```python
from build123d import *

# Parameters (mm, degrees)
F1_DEPTH = 1524
F3_DEPTH = 25.4
F5_DEPTH = 25.4


with BuildPart() as f1:
    # F0 (on Front) → F1 (new body)
    with BuildSketch(Plane.XZ):
        Polygon((-50.705169, 29.967905), (-53.880169, 29.967905), (-53.880169, -14.482095), (-9.430169, -14.482095), (-9.430169, -11.307095), (-50.705169, -11.307095), align=None)
    extrude(amount=F1_DEPTH)

    # F2 (on face) → F3 (cut)
    with BuildSketch(Plane.XY.offset(-11.307095)):
        Polygon((-50.705169, 0), (-9.430169, -41.340452), (-9.430169, 0), align=None)
    extrude(amount=-F3_DEPTH, mode=Mode.SUBTRACT)

    # F4 (on face) → F5 (cut)
    with BuildSketch(Plane.XY.offset(-11.307095)):
        Polygon((-9.430169, -1524), (-9.430169, -1482.725), (-50.705169, -1524), align=None)
    extrude(amount=-F5_DEPTH, mode=Mode.SUBTRACT)


solid = f1.part
```
Here's how the part is built. I have some questions about the finished solid (model axes, mm). A direction names the side the tool comes from. Round coordinates to 2 decimals unless told otherwise and drop trailing zeros. Loops run counter-clockwise (first coordinate to the right, second up) from the corner with the lowest first, then second, coordinate; pieces in that order, holes last.
1. Suppose I cut it at A-A, the plane y = -649. Please give me the cut outline in (x, z).
Answers:
outline: (-53.88, -14.48) - (-9.43, -14.48) - (-9.43, -11.31) - (-50.71, -11.31) - (-50.71, 29.97) - (-53.88, 29.97) - close
2. Suppose I cut it at C-C, the plane x = -21. Please give me the cut outline in (y, z), and give its area (3 significant figures).
Answers:
outline: (-1494.29, -14.48) - (-29.75, -14.48) - (-29.75, -11.31) - (-1494.29, -11.31) - close
area: 4,650 mm2
3. For faces 1 (the face through (-29.779, -1503.074, -12.872)), 2 (the face through (-50.705, -751, 9)), which set-ups out of +Z, -Z, +X, -X, +Y, -Y let a thin tool reach every point of the face, with its end or its side?
Answers:
face 1: +Z, -Z, +X, -Y
face 2: +Z, +X, +Y, -Y
4. Will these pins go through, and if not, where does the flat tip stop? pin 1 (12 mm diameter, centred on x = -19.5, y = -829.5, fed in from +Z); pin 2 (1 mm diameter, centred on y = -265, z = 7.5, fed in from +X).
Answers:
pin 1: stops at z = -11.31
pin 2: stops at x = -50.71
5. Suppose I cut it at B-B, the plane z = 10. Please give me the cut outline in (x, y).
Answers:
outline: (-53.88, -1524) - (-50.71, -1524) - (-50.71, 0) - (-53.88, 0) - close
6. If I drill on probe 1 along Z at (x, y) = (-43, -573.5); probe 2 along X at (y, z) = (-496.5, -11), over which ranges is the centre line in solid material (lowest first)?
Answers:
probe 1: z = -14.48 to -11.31
probe 2: x = -53.88 to -50.71
